Could you check a few things on this model? Use its own coordinates, in mm. A direction names the side the tool comes from. Round coordinates to 2 decimals unless told otherwise and drop trailing zeros. Loops run counter-clockwise (first coordinate to the right, second up) from the corner with the lowest first, then second, coordinate; pieces in that order, holes last. Notation, with made-up numbers: (-8, 21.5) -> (49, 21.5) arc R30 cw to (49, 54.5) -> close; hole circle Ø1 at (43.25, -11). An arc over 180 degrees is marked (long way). One line per item, written item: value.
```python
from build123d import *

# Parameters (mm, degrees)
F3_DEPTH       = 16.05
F4_W           = 5.4241176695
F4_H           = 3.5927895224
F5_DEPTH       = 25
F5_DEPTH_BACK  = 25
F6_T1_DEPTH    = 38.39224199
F8_DEPTH       = 8.025
F8_DEPTH_BACK  = 8.025
F9_T1_DEPTH    = 21.0152154422
F11_W          = 7.7522003338
F11_H          = 3
F12_DEPTH      = 11
F12_DEPTH_BACK = 11
F13_W          = 16.5
F13_H          = 2
F14_DEPTH      = 25
F15_R          = 1
F16_T1_DEPTH   = 22.3322108151
F17_T3_ANGLE   = 128.6137584612
F17_T6_ANGLE   = 128.6137584612
F17_T9_ANGLE   = 166.6195765903
F17_T12_ANGLE  = 166.6195765903
F17_T15_ANGLE  = 208.6372867238
F17_T18_ANGLE  = 208.6372867238
F17_T21_DEPTH  = 5.5
F17_T24_DEPTH  = 5.5
F18_R          = 2
F19_R          = 3


# Not quite as in the source:
# - a fillet or chamfer that OpenCascade refuses, or shapes differently, is made with other operations: its cross-section is extruded or revolved along the edge and cut away or added


with BuildPart() as f3:
    # F2 (on line) → F3 (new body)
    with BuildSketch(Plane.YZ.offset(-8.025)):
        with BuildLine():
            Line((30.8775485963, 0), (34.1775485963, 0))
            ThreePointArc((34.1775485963, 0), (25.0275485963, 9.15), (15.8775485963, 0))
            Line((15.8775485963, 0), (19.1775485963, 0))
            ThreePointArc((19.1775485963, 0), (25.0275485963, 5.85), (30.8775485963, 0))
        make_face()
    extrude(amount=F3_DEPTH)

    # F4 (on Right) → F5 (cut, two sides)
    with BuildSketch(Plane.YZ) as f5_sk:
        with Locations((17.9089335725, 1.7963947612)):
            Rectangle(F4_W, F4_H)
    extrude(amount=-F5_DEPTH, mode=Mode.SUBTRACT)
    extrude(f5_sk.sketch, amount=F5_DEPTH_BACK, mode=Mode.SUBTRACT)

    # F6: fillet of radius 2 on 1 edges, made by hand

    # F6_s2 → F6_t1 (cut)
    with BuildSketch(Plane.YZ.offset(-19.196120995)):
        with BuildLine():
            ThreePointArc((19.3173332992, 7.1495413322), (18.6537711345, 4.9990791235), (20.4108004498, 3.5927895224))
            Line((20.4108004498, 3.5927895224), (16.6124215356, 3.5927895224))
            ThreePointArc((16.6124215356, 3.5927895224), (17.7444211746, 5.5388225246), (19.3173332992, 7.1495413322))
        make_face()
    extrude(amount=F6_T1_DEPTH, mode=Mode.SUBTRACT)

    # F7 (on Right) → F8 (join, two sides)
    with BuildSketch(Plane.YZ) as f8_sk:
        Polygon((34.1775485963, 0), (27.0130820572, 0), (23.9856019616, 0), (10.1775485963, 0), (10.1775485963, -3), (34.1775485963, -3), align=None)
        Polygon((23.9856019616, 0), (27.0130820572, 0), (27.0130820572, 2.18), (27.5856019616, 2.18), (27.5856019616, 3.0622484628), (23.9856019616, 3.0622484628), (23.9856019616, 2.18), align=None)
    extrude(amount=F8_DEPTH)
    extrude(f8_sk.sketch, amount=-F8_DEPTH_BACK)

    # F9: fillet of radius 1 on 1 edges, made by hand

    # F9_s2 → F9_t1 (cut)
    with BuildSketch(Plane.YZ.offset(-10.5076077211)):
        with BuildLine():
            ThreePointArc((27.5856019616, 2.18), (27.2567307119, 2.8098284041), (26.5925588732, 3.0622484628))
            Line((26.5925588732, 3.0622484628), (27.5856019616, 3.0622484628))
            Line((27.5856019616, 3.0622484628), (27.5856019616, 2.18))
        make_face()
    extrude(amount=F9_T1_DEPTH, mode=Mode.SUBTRACT)

    # F10: union 

    # F11 (on Right) → F12 (join, two sides)
    with BuildSketch(Plane.YZ) as f12_sk:
        with Locations((14.0536487631, -1.5)):
            Rectangle(F11_W, F11_H)
    extrude(amount=F12_DEPTH)
    extrude(f12_sk.sketch, amount=-F12_DEPTH_BACK)

    # F13 (on Top) → F14 (cut)
    with BuildSketch(Plane.XY):
        with Locations((0, 14.1775485963)):
            Rectangle(F13_W, F13_H)
    extrude(amount=-F14_DEPTH, mode=Mode.SUBTRACT)

    # F15
    f15_edges = [f3.edges().sort_by_distance(p)[0] for p in [
        (0, 13.177549, -3),
        (0, 13.177549, 0),
    ]]
    fillet(f15_edges, radius=F15_R)

    # F16: fillet of radius 4 on 2 edges, made by hand

    # F16_s2 → F16_t1 (cut)
    with BuildSketch(Plane.XY.offset(-12.6661054076)):
        with BuildLine():
            ThreePointArc((-8.025, 17.92974893), (-10.1701734968, 16.5025689505), (-11, 14.063306767))
            Line((-11, 14.063306767), (-11, 17.92974893))
            Line((-11, 17.92974893), (-8.025, 17.92974893))
        make_face()
        with BuildLine():
            ThreePointArc((8.025, 17.92974893), (10.1701734968, 16.5025689505), (11, 14.063306767))
            Line((11, 14.063306767), (11, 17.92974893))
            Line((11, 17.92974893), (8.025, 17.92974893))
        make_face()
    extrude(amount=F16_T1_DEPTH, mode=Mode.SUBTRACT)

    # F17: fillet of radius 1 on 8 edges, made by hand


with BuildPart() as f17_tool1:
    # F17_s2 → F17_t3 (revolve)
    with BuildSketch(Plane.XY):
        with BuildLine():
            ThreePointArc((-7.025, 34.1775485963), (-7.7321067812, 33.8846553774), (-8.025, 33.1775485963))
            Line((-8.025, 33.1775485963), (-8.025, 34.1775485963))
            Line((-8.025, 34.1775485963), (-7.025, 34.1775485963))
        make_face()
    revolve(axis=Axis((-8.025, 25.0275485963, 0), (1, 0, 0)), revolution_arc=F17_T3_ANGLE)


with BuildPart() as f17_tool4:
    # F17_s5 → F17_t6 (revolve)
    with BuildSketch(Plane.XY):
        with BuildLine():
            ThreePointArc((7.025, 34.1775485963), (7.7321067812, 33.8846553774), (8.025, 33.1775485963))
            Line((8.025, 33.1775485963), (8.025, 34.1775485963))
            Line((8.025, 34.1775485963), (7.025, 34.1775485963))
        make_face()
    revolve(axis=Axis((8.025, 25.0275485963, 0), (1, 0, 0)), revolution_arc=F17_T6_ANGLE)


with BuildPart() as f17_tool7:
    # F17_s8 → F17_t9 (revolve)
    with BuildSketch(Plane(origin=(0, 1.3403038382, 5.634545684), x_dir=(1, 0, 0), z_dir=(0, -0.2314155158, -0.9728550041))):
        with BuildLine():
            ThreePointArc((-7.025, -18.4981758925), (-7.7321067812, -18.2052826737), (-8.025, -17.4981758925))
            Line((-8.025, -17.4981758925), (-8.025, -18.4981758925))
            Line((-8.025, -18.4981758925), (-7.025, -18.4981758925))
        make_face()
    revolve(axis=Axis((-8.025, 25.0275485963, 0), (-1, 0, 0)), revolution_arc=F17_T9_ANGLE)


with BuildPart() as f17_tool10:
    # F17_s11 → F17_t12 (revolve)
    with BuildSketch(Plane(origin=(0, 1.3403038382, 5.634545684), x_dir=(1, 0, 0), z_dir=(0, -0.2314155158, -0.9728550041))):
        with BuildLine():
            ThreePointArc((7.025, -18.4981758925), (7.7321067812, -18.2052826737), (8.025, -17.4981758925))
            Line((8.025, -17.4981758925), (8.025, -18.4981758925))
            Line((8.025, -18.4981758925), (7.025, -18.4981758925))
        make_face()
    revolve(axis=Axis((8.025, 25.0275485963, 0), (-1, 0, 0)), revolution_arc=F17_T12_ANGLE)


with BuildPart() as f17_tool13:
    # F17_s14 → F17_t15 (revolve)
    with BuildSketch(Plane(origin=(0, 5.0675252641, 12.0852942927), x_dir=(1, 0, 0), z_dir=(0, 0.3866941389, 0.9222080259))):
        with BuildLine():
            ThreePointArc((-7.025, 18.8052566142), (-7.7321067812, 18.5123633954), (-8.025, 17.8052566142))
            Line((-8.025, 17.8052566142), (-8.025, 18.8052566142))
            Line((-8.025, 18.8052566142), (-7.025, 18.8052566142))
        make_face()
    revolve(axis=Axis((-8.025, 20.5654677903, 5.5868000574), (-1, 0, 0)), revolution_arc=F17_T15_ANGLE)


with BuildPart() as f17_tool16:
    # F17_s17 → F17_t18 (revolve)
    with BuildSketch(Plane(origin=(0, 5.0675252641, 12.0852942927), x_dir=(1, 0, 0), z_dir=(0, 0.3866941389, 0.9222080259))):
        with BuildLine():
            ThreePointArc((7.025, 18.8052566142), (7.7321067812, 18.5123633954), (8.025, 17.8052566142))
            Line((8.025, 17.8052566142), (8.025, 18.8052566142))
            Line((8.025, 18.8052566142), (7.025, 18.8052566142))
        make_face()
    revolve(axis=Axis((8.025, 20.5654677903, 5.5868000574), (-1, 0, 0)), revolution_arc=F17_T18_ANGLE)


with BuildPart() as f17_tool19:
    # F17_s20 → F17_t21 (new body)
    with BuildSketch(Plane.XY.offset(-5.5)):
        with BuildLine():
            ThreePointArc((7.025, 34.1775485963), (7.7321067812, 33.8846553774), (8.025, 33.1775485963))
            Line((8.025, 33.1775485963), (8.025, 34.1775485963))
            Line((8.025, 34.1775485963), (7.025, 34.1775485963))
        make_face()
    extrude(amount=F17_T21_DEPTH)


with BuildPart() as f17_tool22:
    # F17_s23 → F17_t24 (new body)
    with BuildSketch(Plane.XY.offset(-5.5)):
        with BuildLine():
            ThreePointArc((-7.025, 34.1775485963), (-7.7321067812, 33.8846553774), (-8.025, 33.1775485963))
            Line((-8.025, 33.1775485963), (-8.025, 34.1775485963))
            Line((-8.025, 34.1775485963), (-7.025, 34.1775485963))
        make_face()
    extrude(amount=F17_T24_DEPTH)


with BuildPart() as f3_1:
    add(f3.part)

    # F17_t25: cut F17_tool1, F17_tool4, F17_tool7, F17_tool10, F17_tool13, F17_tool16, F17_tool19, F17_tool22
    add([f17_tool1.part, f17_tool4.part, f17_tool7.part, f17_tool10.part, f17_tool13.part, f17_tool16.part, f17_tool19.part, f17_tool22.part], mode=Mode.SUBTRACT)

    # F18
    f18_edges = [f3_1.edges().sort_by_distance(p)[0] for p in [
        (-11, 10.177549, -1.5),
        (11, 10.177549, -1.5),
    ]]
    fillet(f18_edges, radius=F18_R)

    # F19
    f19_edges = [f3_1.edges().sort_by_distance(p)[0] for p in [
        (-8.025, 17.929749, -1.5),
        (8.025, 17.929749, -1.5),
    ]]
    fillet(f19_edges, radius=F19_R)


solid = f3_1.part
```
(1) Imagine slicing it at B-B on y = 12.5. Write out the boundary of the cut face in (x, z).
Results below:
outline: (-11, -3) -> (-8.25, -3) -> (-8.25, -2.95) -> (8.25, -2.95) -> (8.25, -3) -> (11, -3) -> (11, 0) -> (8.25, 0) -> (8.25, -0.05) -> (-8.25, -0.05) -> (-8.25, 0) -> (-11, 0) -> close
(2) Please list where these lines run through material, in increasing order: L1, parallel to Y at x = -0.5, z = -1.25; L2, parallel to X at y = 26.75, z = 1.75 (3 decimals); L3, parallel to Y at x = -7.75, z = 5.5.
Results below:
L1: y = 10.18 to 13.18, 15.18 to 34.18
L2: x = -8.025 to 8.025
L3: y = 18.88 to 22.25, 27.8 to 31.95
(3) Imagine slicing it at C-C on y = 17.75. Write out the boundary of the cut face in (x, z), then the cut area to 3 significant figures.
Results below:
outline: (-8.83, -3) -> (8.83, -3) -> (8.83, 0) -> (-8.83, 0) -> close
area: 53.0 mm²
(4) Imagine slicing it at A-A on x = -5.25. Write out the boundary of the cut face in (y, z), then the cut area to 3 significant figures.
Results below:
outline: (10.18, -3) -> (12.18, -3) arc R1 ccw to (13.18, -2) -> (13.18, -1) arc R1 ccw to (12.18, 0) -> (10.18, 0) -> close; (15.18, -3) -> (34.18, -3) -> (34.18, 0) arc R9.15 ccw to (19.32, 7.15) arc R2 ccw to (20.41, 3.59) arc R5.85 cw to (30.88, 0) -> (27.01, 0) -> (27.01, 2.18) -> (27.59, 2.18) arc R1 ccw to (26.59, 3.06) -> (23.99, 3.06) -> (23.99, 0) -> (15.18, 0) -> close
area: 136 mm²
(5) For pin 1 Ø2 at (y, z) = (23, 7) entering from +X (3 decimals); pin 2 Ø3 at (x, y) = (2, 29) entering from +Z; pin 3 Ø1.1 at (x, y) = (-7.5, 31.5) entering from +Z; pin 4 Ø1.5 at (y, z) = (17.5, 7) entering from +X, each with a flat end and sliding along its axis, tell me the tip position at first contact or that it passes through.
Results below:
pin 1: stops at x = 8.025
pin 2: stops at z = 8.81
pin 3: stops at z = 6.89
pin 4: passes through
(6) On a 3-axis mill with a long thin cutter (end or side, diameter ignored), from which of +Z, -Z, +X, -X, +Y, -Y can I reach the whole of each face in a straight line? I mean faces 5 (the face through (0, 15.178, -1)), 6 (the face through (-8.025, 26, 1)), 7 (the face through (0.12, 12.89, -0.3)). Say none if no direction works.
Results below:
face 5: +Z, -Z
face 6: +Z, -Z, -X, +Y
face 7: +Z
(7) We'd pull the mould along Y, two halves only. Please class faces 1 (the face through (0, 27.013, 1)), 2 (the face through (-7.724, 33.892, -1.521)), 3 (the face through (0, 10.178, -1)), 4 (the face through (0, 17, 0)): +Y half, -Y half, draft (parallel to the pull), parting line (faces both ways), or undercut.
Results below:
face 1: undercut
face 2: +Y half
face 3: -Y half
face 4: draft
